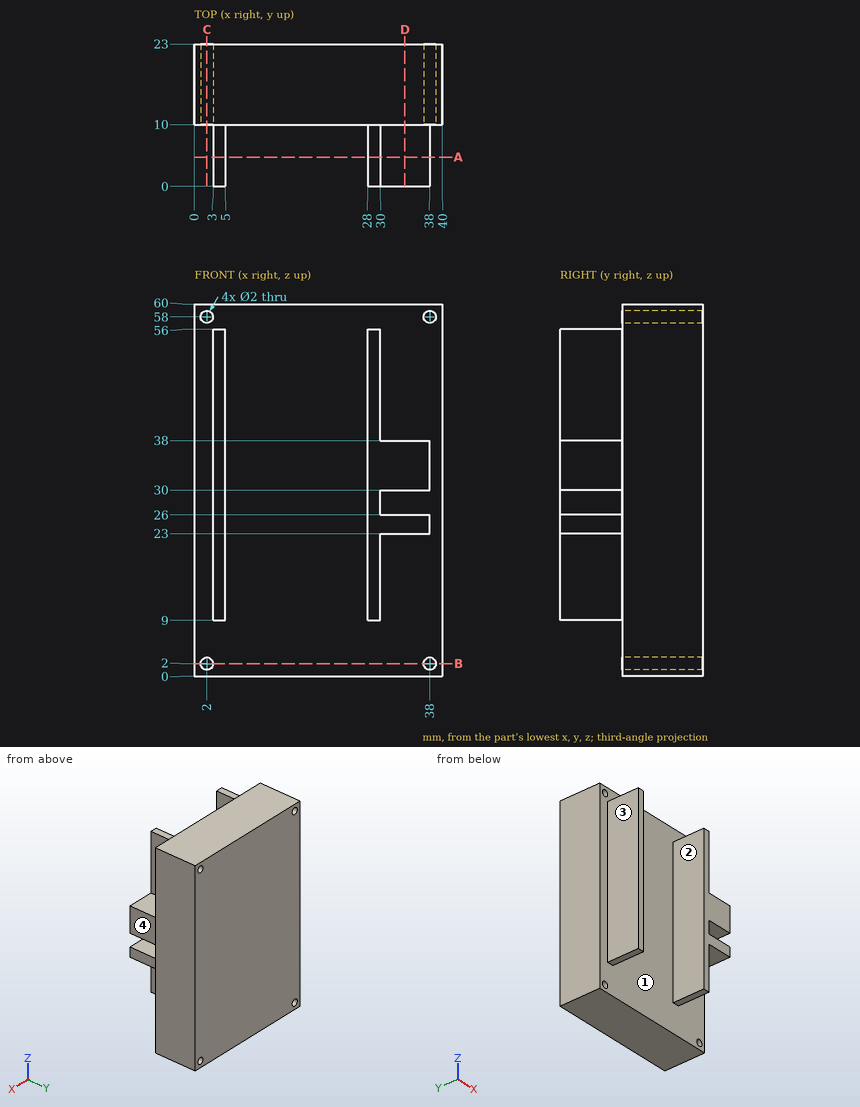
Answer from the drawing. Dimensions are ordinates in mm from the lowest x, y and z of the part. Give positions to 0.01 mm unless a question says otherwise; leave off trailing zeros. Order: outer loops, then holes, each group sorted by start corner. A loop starts at its lowest first (then second) coordinate and runs counter-clockwise, first axis right, second up. Notation, with made-up numbers: (50.5, 72.5) - (86.5, 72.5) arc R25 cw to (86.5, 93.5) - close; hole circle Ø4 at (64, -11). An arc over 180 degrees is marked (long way). Use one line per item in the form item = value.
1) Find section C-C on x = 2. Determine the outline of the cut face in (y, z), and give its area (3 significant figures).
Verdict:
outline = (10, 0) - (23, 0) - (23, 1) - (10, 1) - close; (10, 3) - (23, 3) - (23, 57) - (10, 57) - close; (10, 59) - (23, 59) - (23, 60) - (10, 60) - close
area = 728 mm^2
2) Find section A-A on y = 4.75. Determine the outline of the cut face in (x, z), and give its area (3 significant figures).
Verdict:
outline = (3, 9) - (5, 9) - (5, 56) - (3, 56) - close; (28, 9) - (30, 9) - (30, 23) - (38, 23) - (38, 26) - (30, 26) - (30, 30) - (38, 30) - (38, 38) - (30, 38) - (30, 56) - (28, 56) - close
area = 276 mm^2
3) Each of these flat-tipped pins is pushed along its axis until it touches: pin 1 (6.5 mm diameter, centred on x = 35, y = 3.5, fed in from +Z); pin 2 (8 mm diameter, centred on y = 4.5, z = 47.5, fed in from +X); pin 3 (5 mm diameter, centred on x = 18.5, z = 47.5, fed in from -Y); pin 4 (2 mm diameter, centred on y = 11, z = 30.5, fed in from -X). Where does it stop, or does it pass through?
Verdict:
pin_1 = 38
pin_2 = 30
pin_3 = 10
pin_4 = 0
4) Find section D-D on x = 34. Determine the outline of the cut face in (y, z).
Verdict:
outline = (0, 23) - (10, 23) - (10, 0) - (23, 0) - (23, 60) - (10, 60) - (10, 38) - (0, 38) - (0, 30) - (10, 30) - (10, 26) - (0, 26) - close
5) Consider probe 1 along X at (y, z) = (13.5, 58); probe 2 along Z at (x, y) = (2, 19.25); probe 3 along X at (y, z) = (7.25, 46.5). Determine where each line is inside the solid, lowest interval first. Write a range as [from, to].
Verdict:
probe_1 = [0, 1], [3, 37], [39, 40]
probe_2 = [0, 1], [3, 57], [59, 60]
probe_3 = [3, 5], [28, 30]
6) Find section B-B on z = 2. Determine the outline of the cut face in (x, y).
Verdict:
outline = (0, 10) - (1, 10) - (1, 23) - (0, 23) - close; (3, 10) - (37, 10) - (37, 23) - (3, 23) - close; (39, 10) - (40, 10) - (40, 23) - (39, 23) - close
7) The mould has two halves that part along X. Classify the marked faces 1, 2, 3 and 4: released by +X, released by -X, zero draft, split by the parting line, or undercut.
Verdict:
face_1 = undercut
face_2 = undercut
face_3 = released by -X
face_4 = released by +X
